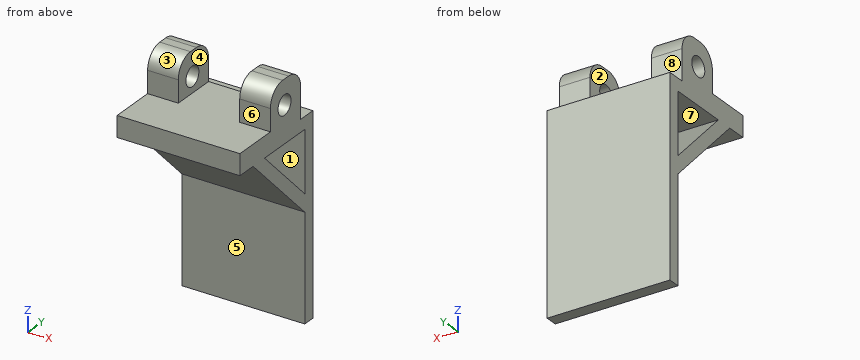
```python
from build123d import *

# Parameters (mm, degrees)
BOSS_EXTRUDE1_DEPTH = 8
SKETCH1_3_W         = 10
SKETCH1_3_H         = 7.5
BOSS_EXTRUDE2_DEPTH = 2
SKETCH2_R           = 1.6
CUT_EXTRUDE1_DEPTH  = 23.808989456
CUT_EXTRUDE3_DEPTH  = 8
FILLET1_R           = 3
BOSS_EXTRUDE3_DEPTH = 3
SKETCH5_W           = 20
SKETCH5_H           = 2
BOSS_EXTRUDE4_DEPTH = 30
BOSS_EXTRUDE5_DEPTH = 20
BOSS_EXTRUDE6_DEPTH = 1.4


with BuildPart() as part:
    # Sketch1 → Boss-Extrude1 (new body)
    with BuildSketch(Plane.XY):
        Polygon((-10, 7.5), (-10, -7.5), (10, -7.5), (10, 7.5), (5, 7.5), (5, 0), (-5, 0), (-5, 7.5), align=None)
    extrude(amount=BOSS_EXTRUDE1_DEPTH)

    # Sketch1<3> → Boss-Extrude2 (add)
    with BuildSketch(Plane.XY):
        Polygon((-10, 7.5), (-10, -7.5), (10, -7.5), (10, 7.5), (5, 7.5), (5, 0), (-5, 0), (-5, 7.5), align=None)
        with Locations((0, 3.75)):
            Rectangle(SKETCH1_3_W, SKETCH1_3_H)
    extrude(amount=-BOSS_EXTRUDE2_DEPTH)

    # Sketch2 → Cut-Extrude1 (cut, through all)
    with BuildSketch(Plane(origin=(10, 0, 0), x_dir=(0, 0, -1), z_dir=(1, 0, 0))):
        with Locations(Location((-4, 3.5, 0), (0, 0, 90))):
            Circle(SKETCH2_R)
    extrude(amount=-CUT_EXTRUDE1_DEPTH, mode=Mode.SUBTRACT)

    # Sketch3 → Cut-Extrude3 (cut)
    with BuildSketch(Plane.XY.offset(8)):
        Polygon((10, -7.5), (10, 0.026252142), (5, 0.026252142), (5, 0), (-5, 0), (-5, 0.026252142), (-10, 0.026252142), (-10, -7.5), align=None)
    extrude(amount=-CUT_EXTRUDE3_DEPTH, mode=Mode.SUBTRACT)

    # Fillet1
    fillet1_edges = [part.edges().sort_by_distance(p)[0] for p in [
        (-7.5, 7.5, 8),
        (7.5, 0.026252142, 8),
        (7.5, 7.5, 8),
        (-7.5, 0.026252142, 8),
    ]]
    fillet(fillet1_edges, radius=FILLET1_R)

    # Sketch4 → Boss-Extrude3 (add)
    with BuildSketch(Plane(origin=(0, 7.5, 0), x_dir=(1, 0, 0), z_dir=(0, 1, 0))):
        Polygon((-5, 0), (5, 0), (10, 0), (10, 2), (-10, 2), (-10, 0), align=None)
    extrude(amount=BOSS_EXTRUDE3_DEPTH)

    # Sketch5 → Boss-Extrude4 (add)
    with BuildSketch(Plane(origin=(0, 0, -2), x_dir=(-1, 0, 0), z_dir=(0, 0, -1))):
        with Locations((0, 9.5)):
            Rectangle(SKETCH5_W, SKETCH5_H)
    extrude(amount=BOSS_EXTRUDE4_DEPTH)

    # Sketch8 → Boss-Extrude5 (add)
    with BuildSketch(Plane(origin=(10, 0, 0), x_dir=(0, 0, -1), z_dir=(1, 0, 0))):
        Polygon((14.757135199, 8.5), (11.934636095, 8.5), (2, -1.434636095), (2, -4.257135199), align=None)
    extrude(amount=-BOSS_EXTRUDE5_DEPTH)

    # Sketch9 → Boss-Extrude6 (add)
    with BuildSketch(Plane.XY):
        Polygon((-5, 7.5), (5, 7.5), (5, 0.026252142), (10, 0.026252142), (10, -7.5), (-10, -7.5), (-10, 0.026252142), (-5, 0.026252142), align=None)
    extrude(amount=BOSS_EXTRUDE6_DEPTH)


solid = part.part
```
Geometry: final body of the model. Coordinates: model frame, mm. Face numbers are marked on the shaded views. A direction names the side the tool comes from. Give positions to 0.01 mm unless a question says otherwise; leave off trailing zeros. Write each loop counter-clockwise with the first axis right and the second up, starting at its lowest first coordinate (ties: lowest second). Pieces come first, ordered by that corner, then holes.
1. Section query B-B, the plane x = 1.5. Return loops of the section in (y, z).
2. Section query C-C, the plane y = 3.5. Return loops of the section in (x, z).
3. Section query A-A, the plane z = 4. Return loops of the section in (x, y).
4. Reachability of the marked faces 4, 5, 6, 7 and 8 from +Z, -Z, +X, -X, +Y, -Y: full face, straight path, thin tool, end or side. Return the list, or none.
5. Draft query along Y for the marked faces 1, 2 and 3. Return one class per face: released by +Y, released by -Y, zero draft, split by the parting line, or undercut.
6. Pin query (flat end, axial travel): P1, Ø3, axis at x = -5, y = 3.5, coming from the -Z side; P2, Ø1.6, axis at x = 2.5, y = -5, coming from the -Z side; P3, Ø1.5, axis at x = 3.5, z = 2, coming from the +Y side. Return the tip coordinate at first contact, or that it passes through.
7. Line query: probe 1 along Z at (x, y) = (-7.9, 3.5); probe 2 along Z at (x, y) = (-6.5, -4.25); probe 3 along Y at (x, z) = (7, -26). Output: solid intervals per line, ascending.
8. Section query D-D, the plane x = 8.75. Return loops of the section in (y, z), then the cut area to 3 significant figures.
Computed:
1. outline: (-7.5, -2) - (-4.26, -2) - (8.5, -14.76) - (8.5, -32) - (10.5, -32) - (10.5, 0) - (7.5, 0) - (7.5, 1.4) - (-7.5, 1.4) - close; hole (-1.43, -2) - (8.5, -11.93) - (8.5, -2) - close
2. outline: (-10, -9.76) - (10, -9.76) - (10, -6.93) - (-10, -6.93) - close; (-10, -2) - (10, -2) - (10, 2.4) - (5, 2.4) - (5, 1.4) - (-5, 1.4) - (-5, 2.4) - (-10, 2.4) - close; (-10, 5.6) - (-5, 5.6) - (-5, 8) - (-10, 8) - close; (5, 5.6) - (10, 5.6) - (10, 8) - (5, 8) - close
3. outline: (-10, 0.03) - (-5, 0.03) - (-5, 1.9) - (-10, 1.9) - close; (-10, 5.1) - (-5, 5.1) - (-5, 7.5) - (-10, 7.5) - close; (5, 0.03) - (10, 0.03) - (10, 1.9) - (5, 1.9) - close; (5, 5.1) - (10, 5.1) - (10, 7.5) - (5, 7.5) - close
4. face 4: +Z, +Y, -Y
4. face 5: -Z, +X, -X, -Y
4. face 6: +Z, +X, -X, -Y
4. face 7: +X, -X
4. face 8: +Z, +X, -X, +Y
5. face 1: undercut
5. face 2: zero draft
5. face 3: released by -Y
6. P1: stops at z = -11.26
6. P2: stops at z = -2.06
6. P3: stops at y = 7.5
7. probe 1: z = -9.76 to -6.93, -2 to 2.4, 5.6 to 8
7. probe 2: z = -2.01 to 1.4
7. probe 3: y = 8.5 to 10.5
8. outline: (-7.5, -2) - (-4.26, -2) - (8.5, -14.76) - (8.5, -32) - (10.5, -32) - (10.5, 0) - (7.5, 0) - (7.5, 5) arc R3 ccw to (4.5, 8) - (3.03, 8) arc R3 ccw to (0.03, 5) - (0.03, 1.4) - (-7.5, 1.4) - close; hole (-1.43, -2) - (8.5, -11.93) - (8.5, -2) - close; hole circle Ø3.2 at (3.5, 4)
8. area: 186 mm2
